Model file for the job. Use its own axes, mm. A direction names the side the tool comes from. Give positions to 0.01 mm unless a question says otherwise; leave off trailing zeros. Write each loop counter-clockwise with the first axis right and the second up, starting at its lowest first coordinate (ties: lowest second). Pieces come first, ordered by that corner, then holes. Notation, with made-up numbers: (54, -4) - (81, -4) arc R10 ccw to (81, 11) - close; hole circle Ø8 at (61.5, 19). An arc over 180 degrees is marked (long way). Use CSV: the item, a comma, the result in double quotes.
from build123d import *

# Parameters (mm, degrees)
SKETCH4_R           = 82.042
BOSS_EXTRUDE2_DEPTH = 0.508
SKETCH5_R           = 69.342
CUT_EXTRUDE5_DEPTH  = 1.508
CUT_EXTRUDE6_DEPTH  = 1.508
CUT_EXTRUDE11_DEPTH = 1.508


with BuildPart() as part:
    # Sketch4 → Boss-Extrude2 (new body)
    with BuildSketch(Plane.XY):
        Circle(SKETCH4_R)
    extrude(amount=BOSS_EXTRUDE2_DEPTH)

    # Sketch5 → Cut-Extrude5 (cut, through all)
    with BuildSketch(Plane.XY.offset(0.508)):
        Circle(SKETCH5_R)
    extrude(amount=-CUT_EXTRUDE5_DEPTH, mode=Mode.SUBTRACT)

    # Sketch6 → Cut-Extrude6 (cut, through all)
    with BuildSketch(Plane.XY.offset(0.508)):
        with BuildLine():
            ThreePointArc((56.845021902, 56.845020591), (50.199631755, 56.845021285), (50.199632296, 50.199631138))
            ThreePointArc((50.199632296, 50.199631138), (65.588979611, 27.167845011), (70.993, 1.03e-06))
            ThreePointArc((70.993, 1.03e-06), (75.692000068, -4.699), (80.391, 1.166e-06))
            ThreePointArc((80.391, 1.166e-06), (74.271599452, 30.764303922), (56.845021902, 56.845020591))
        make_face()
        with BuildLine():
            ThreePointArc((56.845020591, -56.845021902), (56.845021285, -50.199631755), (50.199631138, -50.199632296))
            ThreePointArc((50.199631138, -50.199632296), (27.167845011, -65.588979611), (1.03e-06, -70.993))
            ThreePointArc((1.03e-06, -70.993), (-4.699, -75.692000068), (1.166e-06, -80.391))
            ThreePointArc((1.166e-06, -80.391), (30.764303922, -74.271599452), (56.845020591, -56.845021902))
        make_face()
        with BuildLine():
            ThreePointArc((-56.845021902, -56.845020591), (-50.199631755, -56.845021285), (-50.199632296, -50.199631138))
            ThreePointArc((-50.199632296, -50.199631138), (-65.588979611, -27.167845011), (-70.993, -1.03e-06))
            ThreePointArc((-70.993, -1.03e-06), (-75.692000068, 4.699), (-80.391, -1.166e-06))
            ThreePointArc((-80.391, -1.166e-06), (-74.271599452, -30.764303922), (-56.845021902, -56.845020591))
        make_face()
        with BuildLine():
            ThreePointArc((-56.845020591, 56.845021902), (-56.845021285, 50.199631755), (-50.199631138, 50.199632296))
            ThreePointArc((-50.199631138, 50.199632296), (-27.167845011, 65.588979611), (-1.03e-06, 70.993))
            ThreePointArc((-1.03e-06, 70.993), (4.699, 75.692000068), (-1.166e-06, 80.391))
            ThreePointArc((-1.166e-06, 80.391), (-30.764303922, 74.271599452), (-56.845020591, 56.845021902))
        make_face()
    extrude(amount=-CUT_EXTRUDE6_DEPTH, mode=Mode.SUBTRACT)

    # Sketch8 → Cut-Extrude11 (cut, through all)
    with BuildSketch(Plane.XY.offset(0.508)):
        Polygon((76.869596069, 30.465791131), (75.89758015, 32.812445144), (74.724253144, 32.326437185), (75.696269062, 29.979783172), align=None)
        Polygon((-30.465791131, 76.869596069), (-32.812445144, 75.89758015), (-32.326437185, 74.724253144), (-29.979783172, 75.696269062), align=None)
        Polygon((-75.89758015, 32.812445144), (-76.869596069, 30.465791131), (-75.696269062, 29.979783172), (-74.724253144, 32.326437185), align=None)
        Polygon((-76.869596069, -30.465791131), (-75.89758015, -32.812445144), (-74.724253144, -32.326437185), (-75.696269062, -29.979783172), align=None)
        Polygon((-32.812445144, -75.89758015), (-30.465791131, -76.869596069), (-29.979783172, -75.696269062), (-32.326437185, -74.724253144), align=None)
        Polygon((30.465791131, -76.869596069), (32.812445144, -75.89758015), (32.326437185, -74.724253144), (29.979783172, -75.696269062), align=None)
        Polygon((75.89758015, -32.812445144), (76.869596069, -30.465791131), (75.696269062, -29.979783172), (74.724253144, -32.326437185), align=None)
        Polygon((32.812445144, 75.89758015), (30.465791131, 76.869596069), (29.979783172, 75.696269062), (32.326437185, 74.724253144), align=None)
    extrude(amount=-CUT_EXTRUDE11_DEPTH, mode=Mode.SUBTRACT)


solid = part.part
(1) Saw through at C-C, the plane z = 0.1. Count the separate pieces of the cut face and the enclosed holes in it, then the cut area to 3 significant figures.
Checked values:
separate pieces,"1"
enclosed holes,"5"
area,"3,510 mm^2"
(2) Saw through at B-B, the plane x = 27. List the corners of the cut face in (y, z), then the cut area to 3 significant figures.
Checked values:
outline,"(-77.47, 0) - (-75.72, 0) - (-75.72, 0.51) - (-77.47, 0.51) - close; (-65.66, 0) - (-63.87, 0) - (-63.87, 0.51) - (-65.66, 0.51) - close; (63.87, 0) - (77.47, 0) - (77.47, 0.51) - (63.87, 0.51) - close"
area,"8.71 mm^2"
(3) Wall check: probe 1 along Y at (x, z) = (12.5, 0.3); probe 2 along Y at (x, z) = (6, 0.45); probe 3 along X at (y, z) = (57, 0.1). Give the ranges that are in metal, low to high. Write a range as [from, to].
Checked values:
probe 1,"y = [-81.08, -79.41], [-69.88, -68.21], [68.21, 81.08]"
probe 2,"y = [-81.82, -80.17], [-70.74, -69.08], [69.08, 81.82]"
probe 3,"x = [-59.01, -56.69], [-42.32, -39.49], [39.49, 50.36], [56.68, 59.01]"
(4) Pull direction Y, two halves, no side cores. Call faces 3 (the face through (50.273, 56.917, 0.258)), 4 (the face through (0.43, 82.04, 0.25)), 5 (the face through (-58.318, -57.705, 0.25)), 6 (the face through (75.6, -4.7, 0.3)): released by +Y, released by -Y, zero draft, split by the parting line, or undercut.
Checked values:
face 3,"undercut"
face 4,"released by +Y"
face 5,"released by -Y"
face 6,"undercut"
(5) Saw through at A-A, the plane y = -64.5. List the corners of the cut face in (x, z).
Checked values:
outline,"(-50.7, 0) - (-25.46, 0) - (-25.46, 0.51) - (-50.7, 0.51) - close; (25.46, 0) - (29.66, 0) - (29.66, 0.51) - (25.46, 0.51) - close; (47.98, 0) - (50.7, 0) - (50.7, 0.51) - (47.98, 0.51) - close"
(6) 3-axis set-ups, long thin cutter, end or side, ignore diameter. For faces 1 (the face through (-0.43, -82.04, 0.25)), 2 (the face through (-74.44, -30.356, 0.258)): which of +Z, -Z, +X, -X, +Y, -Y reach the whole face in a straight line?
Checked values:
face 1,"+Z, -Z, -Y"
face 2,"+Z, -Z"
